Could you check a few things on this model? Use its own coordinates, in mm. Face numbers are marked on the shaded views. A direction names the side the tool comes from. Give positions to 0.01 mm unless a question says otherwise; leave off trailing zeros. Order: outer loops, then holes, each group sorted by start corner. A loop starts at its lowest first (then second) coordinate and runs counter-clockwise, first axis right, second up. Notation, with made-up numbers: (78, 86) -> (82, 86) arc R13 ccw to (82, 102) -> close; hole circle Ø10 at (-8.75, -11). An arc over 180 degrees is marked (long way). Use one line per item in the form item = value. Start each with the question number.
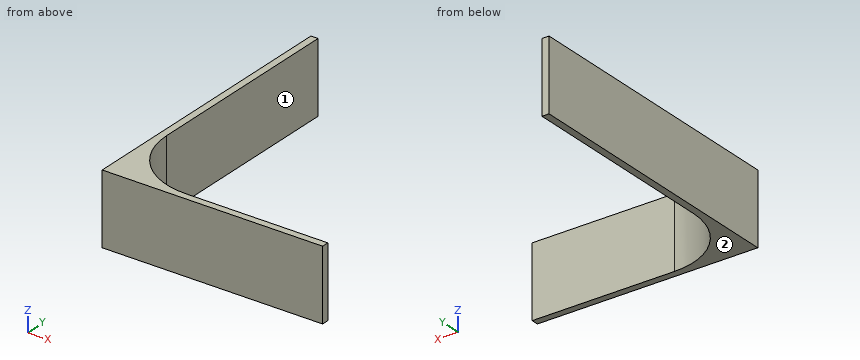
from build123d import *

# Parameters (mm, degrees)
SKETCH1_W           = 30
SKETCH1_H           = 10
BOSS_EXTRUDE1_DEPTH = 1
SKETCH4_W           = 10
SKETCH4_H           = 40
BOSS_EXTRUDE2_DEPTH = 1
FILLET2_R           = 10


with BuildPart() as part:
    # Sketch1 → Boss-Extrude1 (new body)
    with BuildSketch(Plane(origin=(0, 0, 0), x_dir=(1, 0, 0), z_dir=(0, 1, 0))):
        with Locations((15, 5)):
            Rectangle(SKETCH1_W, SKETCH1_H)
    extrude(amount=BOSS_EXTRUDE1_DEPTH)

    # Sketch4 → Boss-Extrude2 (add)
    with BuildSketch(Plane(origin=(0, 0, 0), x_dir=(0, 0, -1), z_dir=(1, 0, 0))):
        with Locations((5, 20)):
            Rectangle(SKETCH4_W, SKETCH4_H)
    extrude(amount=-BOSS_EXTRUDE2_DEPTH)

    # Fillet2
    fillet2_edges = [part.edges().sort_by_distance(p)[0] for p in [
        (0, 1, -5),
    ]]
    fillet(fillet2_edges, radius=FILLET2_R)


solid = part.part
(1) Which directions (+Z, -Z, +X, -X, +Y, -Y) give clear straight access to the entire face, cutting with the end or side of a thin tool? Please do the marked faces 1 and 2.
(2) Imagine slicing it at A-A (z = -3). Write out the boundary of the cut face in (x, y).
(3) Imagine slicing it at C-C (y = 16). Write out the boundary of the cut face in (x, z), plus the area to 3 significant figures.
(4) Imagine slicing it at B-B (x = 11). Write out the boundary of the cut face in (y, z).
(5) Please list where these lines run through material, in increasing order: probe 1 along Y at (x, z) = (28.5, -8.75); probe 2 along X at (y, z) = (21.5, -6.25); probe 3 along X at (y, z) = (9, -8.75).
(6) I'm going to push flat-ended pins straight in: pin 1 Ø3 at (y, z) = (26.5, -6) entering from +X; pin 2 Ø2 at (x, z) = (8, -1) entering from +Y; pin 3 Ø3 at (x, z) = (22, -3) entering from +Y. Where does each tip first touch, or does it pass through?
Calculated:
q1.face_1 = +Z, -Z, +X, +Y
q1.face_2 = -Z, +X, -X, +Y, -Y
q2.outline = (-1, 0) -> (30, 0) -> (30, 1) -> (10, 1) arc R10 cw to (0, 11) -> (0, 40) -> (-1, 40) -> close
q3.outline = (-1, -10) -> (0, -10) -> (0, 0) -> (-1, 0) -> close
q3.area = 10.0 mm2
q4.outline = (0, -10) -> (1, -10) -> (1, 0) -> (0, 0) -> close
q5.probe_1 = 0 to 1
q5.probe_2 = -1 to 0
q5.probe_3 = -1 to 0.2
q6.pin_1 = 0
q6.pin_2 = 1.46
q6.pin_3 = 1
